Read the model definition and answer for the solid it produces. Units are mm, in the model's axes. Face numbers are marked on the shaded views. Round coordinates to 2 decimals unless told otherwise and drop trailing zeros. Order: outer loops, then holes, each group sorted by start corner. A loop starts at its lowest first (then second) coordinate and runs counter-clockwise, first axis right, second up.
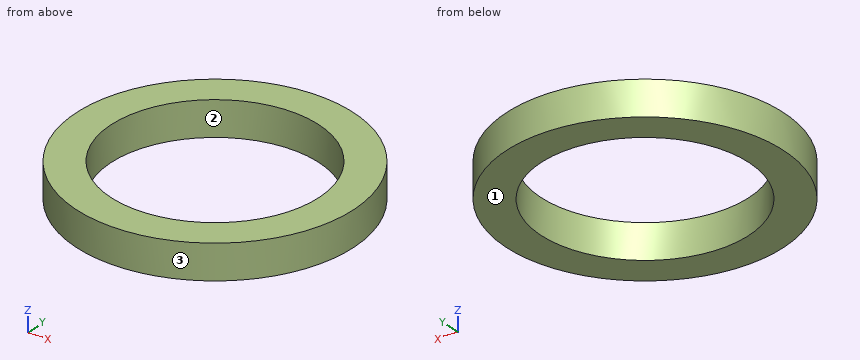
from build123d import *

# Parameters (mm, degrees)
CYLINDER154_R     = 7.14375
CYLINDER154_DEPTH = 2.38125
CYLINDER155_R     = 9.525
CYLINDER155_DEPTH = 2.38125


with BuildPart() as cylinder008:
    # Cylinder154 → Cylinder154 (new body)
    with BuildSketch(Plane.XY.offset(-21)):
        Circle(CYLINDER154_R)
    extrude(amount=CYLINDER154_DEPTH)


with BuildPart() as cut019:
    # Cylinder155 → Cylinder155 (new body)
    with BuildSketch(Plane.XY.offset(-21)):
        Circle(CYLINDER155_R)
    extrude(amount=CYLINDER155_DEPTH)

    # Cut019: cut Cylinder008
    add(cylinder008.part, mode=Mode.SUBTRACT)


solid = cut019.part
Q1. A cutting plane is placed at B-B, the plane y = 5. Give the vertices of the cut face in (x, z), plus the area to 3 significant figures.
Outcome:
outline: (-8.11, -21) - (-5.1, -21) - (-5.1, -18.62) - (-8.11, -18.62) - close; (5.1, -21) - (8.11, -21) - (8.11, -18.62) - (5.1, -18.62) - close
area: 14.3 mm2
Q2. Flat-ended cylindrical pins translate along their axes: pin 1 (1 mm diameter, centred on x = -1, z = -20.5, fed in from +Y); pin 2 (5 mm diameter, centred on x = -3, y = 1, fed in from -Z). Find the tip coordinate at first contact, or state that the pin passes through.
Outcome:
pin 1: stops at y = 9.51
pin 2: passes through
Q3. For a pull along X with two mould halves and no side action, classify the marked faces 1, 2 and 3 as released by +X, released by -X, zero draft, split by the parting line, or undercut.
Outcome:
face 1: zero draft
face 2: undercut
face 3: split by the parting line
Q4. Straight lines are drawn through the part: probe 1 along Y at (x, z) = (-6.25, -18.85); probe 2 along Y at (x, z) = (2.75, -19.3); probe 3 along X at (y, z) = (6, -20.8). For each, find the intervals that lie inside material, in ascending order.
Outcome:
probe 1: y = -7.19 to -3.46, 3.46 to 7.19
probe 2: y = -9.12 to -6.59, 6.59 to 9.12
probe 3: x = -7.4 to -3.88, 3.88 to 7.4
Q5. A cutting plane is placed at A-A, the plane x = 0. Give the vertices of the cut face in (y, z) (3 decimals), plus the area to 3 significant figures.
Outcome:
outline: (-9.525, -21) - (-7.144, -21) - (-7.144, -18.619) - (-9.525, -18.619) - close; (7.144, -21) - (9.525, -21) - (9.525, -18.619) - (7.144, -18.619) - close
area: 11.3 mm2
